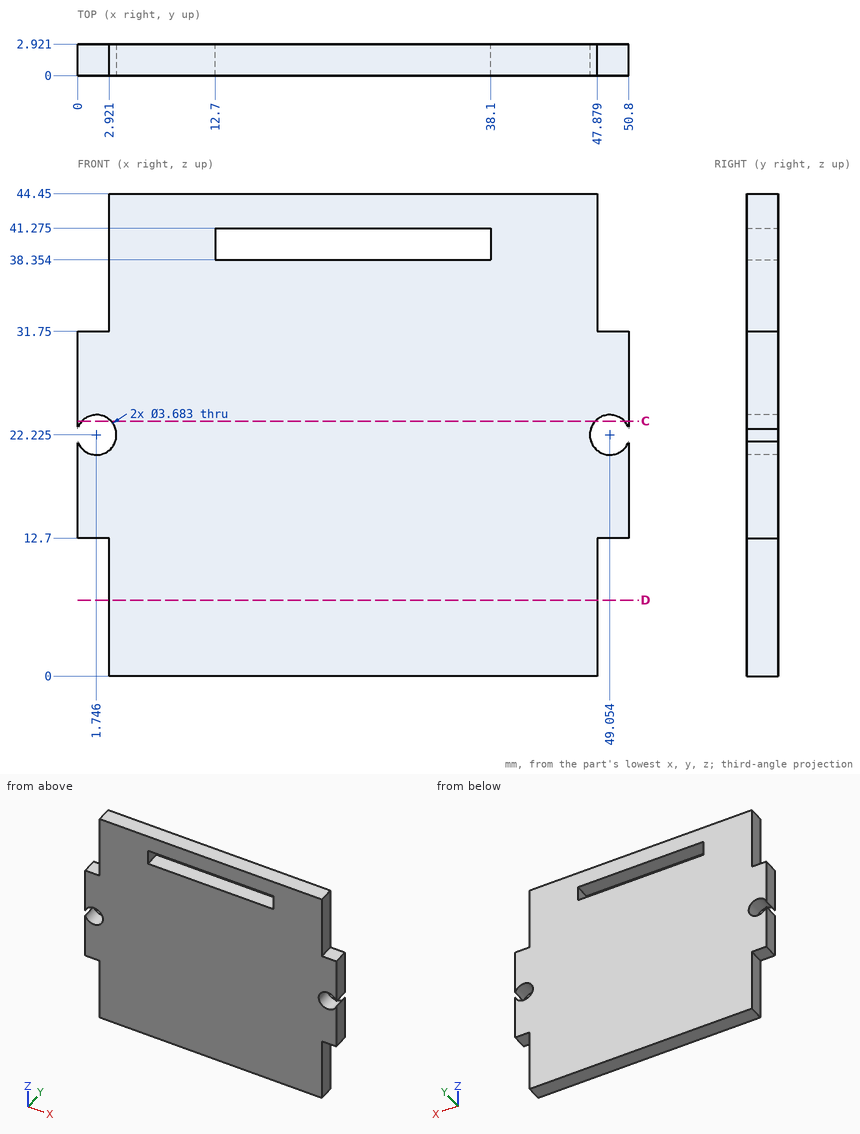
Part print with two shaded views. Sizes in mm from the minimum x, y, z corner. Coordinates: 2 decimals unless noted, no trailing zeros. Order: outer loops, then holes, each group sorted by start corner. A loop starts at its lowest first (then second) coordinate and runs counter-clockwise, first axis right, second up. Notation, with made-up numbers: (62.5, -8.5) - (97.5, -8.5) arc R27 ccw to (97.5, 25.5) - close; hole circle Ø1 at (18.25, -27). An arc over 180 degrees is marked (long way). Write item = value, one per line. Start each with the question number.
1) Saw through at D-D on z = 7. Write the cut outline in (x, y).
2) Saw through at C-C on z = 23.5. Write the cut outline in (x, y) (1 decimal), then the cut area to 3 significant figures.
3) Wall check: line 1 along X through (y, z) = (0.5, 8.5); line 2 along X through (y, z) = (0.7, 21). Give the ranges that are in metal, low to high. Write a range as from..to.
4) Flat gauge pins, fed straight in: pin 1 Ø1.5 at (y, z) = (2, 39.5) entering from +X; pin 2 Ø1.5 at (y, z) = (1, 39.5) entering from -X; pin 3 Ø1.5 at (x, y) = (50, 1.5) entering from -Z. Where does each tip first touch, or does it go through?
From the geometry:
q1.outline = (2.92, 0) - (47.88, 0) - (47.88, 2.92) - (2.92, 2.92) - close
q2.outline = (0, 0) - (0.4, 0) - (0.4, 2.9) - (0, 2.9) - close; (3.1, 0) - (47.7, 0) - (47.7, 2.9) - (3.1, 2.9) - close; (50.4, 0) - (50.8, 0) - (50.8, 2.9) - (50.4, 2.9) - close
q2.area = 133 mm^2
q3.line_1 = 2.92..47.88
q3.line_2 = 0..0.37, 3.12..47.68, 50.43..50.8
q4.pin_1 = 47.88
q4.pin_2 = 2.92
q4.pin_3 = 12.7
